Geometry check sheet. Reference: the model listing, model coordinates, mm. Coordinates: 2 decimals unless noted, no trailing zeros. Write each loop counter-clockwise with the first axis right and the second up, starting at its lowest first coordinate (ties: lowest second). Pieces come first, ordered by that corner, then holes. Notation, with made-up numbers: M 64.25,41 L 103.25,41 A29 ccw 103.25,65 Z; hole C -18,79 d6. An arc over 180 degrees is marked long. Put each result on its own line as item: value. Start each with the question number.
1) Cross-section at A-A on y = 0.55. Record the cut outline in (x, z) (3 decimals), plus the area to 3 significant figures.
2) Gauge pin test, flat end, axial feed: pin 1 (1 mm diameter, centred on y = 0.5, z = -0.5, fed in from +X). Record the tip position at first contact, or that the pin passes through.
3) Scan lines: line 1 along X through (y, z) = (0.8, -2.1) (3 decimals); line 2 along Y through (x, z) = (14.5, -1.9); line 3 along Y through (x, z) = (15, -0.5). Record each from-to range of solid material in increasing order.
from build123d import *

# Parameters (mm, degrees)
SKETCH1_W             = 34.75
SKETCH1_H             = 5
BOSS_EXTRUDE1_DEPTH   = 2.5
F_1_0MM_DOWEL_HOLE1_D = 2.005
SKETCH15_RX           = 6.5
SKETCH15_RY           = 1.5
CUT_EXTRUDE1_DEPTH    = 10
FILLET1_START         = -3
FILLET1_DEPTH         = 6
FILLET2_R             = 3


with BuildPart() as part:
    # Sketch1 → Boss-Extrude1 (new body)
    with BuildSketch(Plane(origin=(0, 0, 0), x_dir=(1, 0, 0), z_dir=(0, 1, 0))):
        Rectangle(SKETCH1_W, SKETCH1_H)
    extrude(amount=BOSS_EXTRUDE1_DEPTH)

    # Ø1.0mm Dowel Hole1 (through all)
    with Locations(Plane.XY.offset(2.5)):
        with Locations((-8.025, 1.25)):
            Hole(F_1_0MM_DOWEL_HOLE1_D / 2)

    # Sketch15 → Cut-Extrude1 (cut)
    with BuildSketch(Plane.XY.offset(2.5)):
        with Locations((-17.375, 2.5)):
            Ellipse(SKETCH15_RX, SKETCH15_RY)
    extrude(amount=-CUT_EXTRUDE1_DEPTH, mode=Mode.SUBTRACT)

    # Fillet1: read off the stored shape, not the designer's step
    # Fillet1 outline → Fillet1 (cut)
    with BuildSketch(Plane.XY.offset(FILLET1_START)):
        with BuildLine():
            ThreePointArc((-10.948655177, 2.274826432), (-10.768220883, 2.440121129), (-10.530958598, 2.5))
            Line((-10.530958598, 2.5), (-10.875, 2.5))
            add(Edge.make_bspline(
                [(-10.948655177, 2.274826432), (-10.875, 2.386771689), (-10.875, 2.5)],
                knots=[6.120582714, 6.120582714, 6.120582714, 6.283185307, 6.283185307, 6.283185307], degree=2, weights=[0.94563875, 0.969680858, 1]))
        make_face()
    extrude(amount=FILLET1_DEPTH, mode=Mode.SUBTRACT)

    # Fillet2
    # the kernel refuses this fillet: 3 mm, written as the material it takes off along each edge
    with BuildSketch(Plane(origin=(17.375, 0, -9.895099729), x_dir=(-1, 0, 0), z_dir=(0, 0, 1))) as fillet2_piece_1:
        with BuildLine():
            CenterArc((2.958039892, -3), FILLET2_R, 90, 80.405931773)
            Line((0, -2.5), (-0.059160798, -2.49))
            ThreePointArc((-0.059160798, -2.49), (-0.06, -1.25), (-0.06, 0))
            Line((-0.06, 0), (0, 0.06))
            Line((0, 0.06), (2.958039892, 0.06))
            Line((2.958039892, 0.06), (2.958039892, 0))
        make_face()
    extrude(amount=19.790199458, mode=Mode.SUBTRACT)


solid = part.part
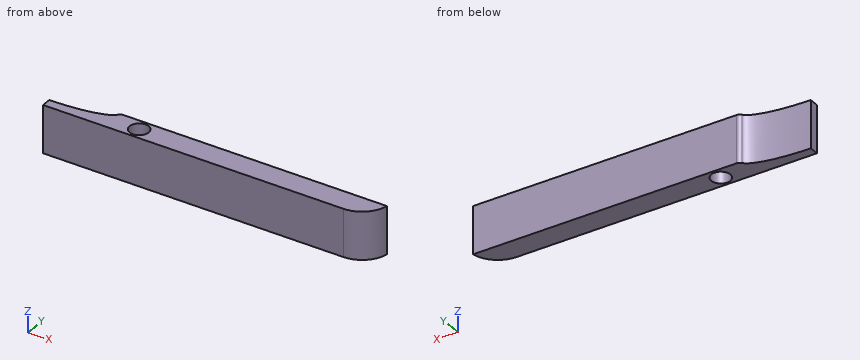
Answer key:
1. outline: M -17.375,-2.5 L -8.743,-2.5 L -8.743,2.5 L -17.375,2.5 Z; M -7.307,-2.5 L 16.148,-2.5 L 16.148,2.5 L -7.307,2.5 Z
1. area: 160 mm²
2. pin 1: stops at x = 16.65
3. line 1: x = -17.375 to -8.921, -7.129 to 16.457
3. line 2: y = 0 to 2.5
3. line 3: y = 0.06 to 2.5
